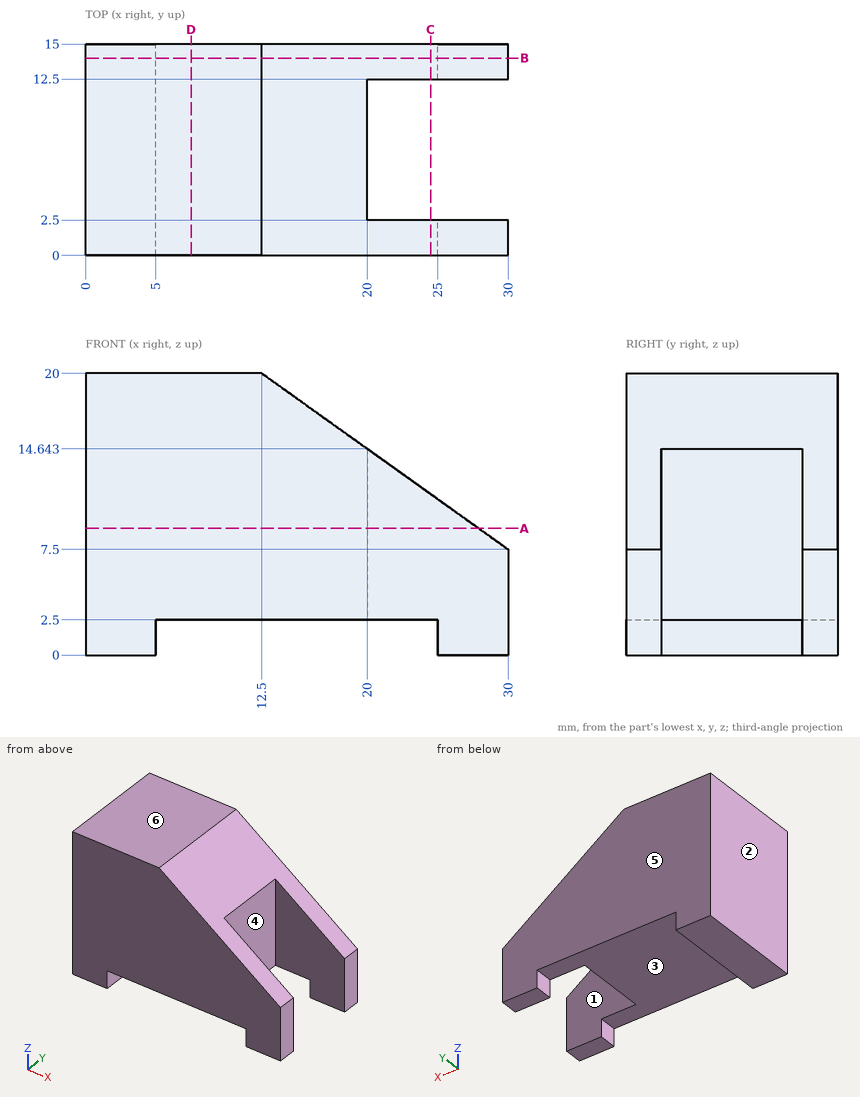
Could you check a few things on this drawing? It's one solid part, dimensions in mm from its lowest x, y, z. A direction names the side the tool comes from. Give positions to 0.01 mm unless a question says otherwise; leave off trailing zeros. Write each loop counter-clockwise with the first axis right and the second up, starting at its lowest first coordinate (ties: lowest second). Pieces come first, ordered by that corner, then holes. Notation, with made-up numbers: M 8.5,23.5 L 28.5,23.5 A30 ccw 28.5,53.5 Z; hole C -25.75,-32 d11. An arc over 180 degrees is marked long. Put each result on its own line as item: value. Start each with the question number.
Item 1: If we section it at B-B, the plane y = 14: Write out the boundary of the cut face in (x, z), then the cut area to 3 significant figures.
Item 2: I need wall thicknesses on L1, parallel to Y at x = 24, z = 3.5; L2, parallel to X at y = 9, z = 7.5; L3, parallel to Z at x = 7.5, y = 10.75. Which ranges of each line are inside material? Lowest first, please. Write a range as from..to.
Item 3: Thinking about a two-plate mould opening in Y: for the marked faces 4, 5 and 6, which applies, +Y half, -Y half, draft (parallel to the pull), parting line (faces both ways), or undercut?
Item 4: If we section it at A-A, the plane z = 9: Write out the boundary of the cut face in (x, y), then the cut area to 4 significant figures.
Item 5: On a 3-axis mill with a long thin cutter (end or side, diameter ignored), from which of +Z, -Z, +X, -X, +Y, -Y can I reach the whole of each face in a straight line? I mean the marked faces 1, 2 and 3. Say none if no direction works.
Item 6: If we section it at C-C, the plane x = 24.5: Write out the boundary of the cut face in (y, z).
Item 7: Will these pins go through, and if not, where does the flat tip stop? pin 1 (8 mm diameter, centred on y = 7, z = 6.5, fed in from +X); pin 2 (6 mm diameter, centred on x = 21.5, y = 11, fed in from +Z); pin 3 (4 mm diameter, centred on x = 7.5, y = 2, fed in from -Z).
Item 8: If we section it at D-D, the plane x = 7.5: Write out the boundary of the cut face in (y, z).
Values:
1. outline: M 0,0 L 5,0 L 5,2.5 L 25,2.5 L 25,0 L 30,0 L 30,7.5 L 12.5,20 L 0,20 Z
1. area: 441 mm²
2. L1: 0..2.5, 12.5..15
2. L2: 0..20
2. L3: 2.5..20
3. face 4: undercut
3. face 5: +Y half
3. face 6: draft
4. outline: M 0,0 L 27.9,0 L 27.9,2.5 L 20,2.5 L 20,12.5 L 27.9,12.5 L 27.9,15 L 0,15 Z
4. area: 339.5 mm²
5. face 1: +Z, -Z, +X
5. face 2: +Z, -Z, -X, +Y, -Y
5. face 3: -Z, +Y, -Y
6. outline: M 0,2.5 L 2.5,2.5 L 2.5,11.43 L 0,11.43 Z; M 12.5,2.5 L 15,2.5 L 15,11.43 L 12.5,11.43 Z
7. pin 1: x = 20
7. pin 2: z = 15.71
7. pin 3: z = 2.5
8. outline: M 0,2.5 L 15,2.5 L 15,20 L 0,20 Z
